Could you check a few things on this model? Use its own coordinates, in mm. A direction names the side the tool comes from. Coordinates: 2 decimals unless noted, no trailing zeros. Loops run counter-clockwise (first coordinate to the right, second up) from the corner with the lowest first, then second, coordinate; pieces in that order, holes last.
from build123d import *

# Parameters (mm, degrees)
SKETCH2_R           = 20.9
SKETCH2_R_2         = 20.4
BOSS_EXTRUDE1_DEPTH = 66
SKETCH3_R           = 20.848686735
BOSS_EXTRUDE2_DEPTH = 0.1
SKETCH4_R           = 8.6
BOSS_EXTRUDE3_DEPTH = 3.5
SKETCH5_R           = 2.4
BOSS_EXTRUDE4_DEPTH = 1.35
SKETCH7_R           = 2.4
CUT_EXTRUDE1_DEPTH  = 76.523969705
CUT_EXTRUDE6_DEPTH  = 73.316111621
CIRPATTERN2_COUNT   = 4


with BuildPart() as part:
    # Sketch2 → Boss-Extrude1 (new body)
    with BuildSketch(Plane(origin=(0, 0, 0), x_dir=(1, 0, 0), z_dir=(0, 1, 0))):
        with Locations(Location((0, 0, 0), (0, 0, 270))):
            Circle(SKETCH2_R)
        with Locations(Location((0, 0, 0), (0, 0, 270))):
            Circle(SKETCH2_R_2, mode=Mode.SUBTRACT)
    extrude(amount=BOSS_EXTRUDE1_DEPTH)

    # Sketch3 → Boss-Extrude2 (add)
    with BuildSketch(Plane(origin=(0, 0, 0), x_dir=(1, 0, 0), z_dir=(0, 1, 0))):
        Circle(SKETCH3_R)
    extrude(amount=BOSS_EXTRUDE2_DEPTH)

    # Sketch4 → Boss-Extrude3 (add)
    with BuildSketch(Plane(origin=(0, 0, 0), x_dir=(1, 0, 0), z_dir=(0, 1, 0))):
        with Locations(Location((0.271248052, 0, 0), (0, 0, 270))):
            Circle(SKETCH4_R)
    extrude(amount=-BOSS_EXTRUDE3_DEPTH)

    # Sketch5 → Boss-Extrude4 (add)
    with BuildSketch(Plane.XZ.offset(3.5)):
        with Locations((0.36166407, 0)):
            Circle(SKETCH5_R)
    extrude(amount=-BOSS_EXTRUDE4_DEPTH)

    # Sketch7 → Cut-Extrude1 (cut, through all)
    with BuildSketch(Plane.XZ.offset(3.5)):
        with Locations(Location((0.271248052, 0, 0), (0, 0, 270))):
            Circle(SKETCH7_R)
    extrude(amount=-CUT_EXTRUDE1_DEPTH, mode=Mode.SUBTRACT)

    # Sketch15 → Cut-Extrude6 (cut, through all)
    with BuildSketch(Plane(origin=(0, 0, 0), x_dir=(0, 0, -1), z_dir=(1, 0, 0))):
        with BuildLine():
            Line((-2.657246102, 51), (9.342753898, 51))
            ThreePointArc((9.342753898, 51), (12.842753898, 47.5), (9.342753898, 44))
            Line((9.342753898, 44), (-2.657246102, 44))
            ThreePointArc((-2.657246102, 44), (-6.157246102, 47.5), (-2.657246102, 51))
        make_face()
    cut_extrude6 = extrude(amount=-CUT_EXTRUDE6_DEPTH, mode=Mode.SUBTRACT)

    # CirPattern2: Cut-Extrude6 ×4 about axis
    cirpattern2_axis = Axis((0, 66, 0), (0, -1, 0))
    for i in range(1, CIRPATTERN2_COUNT):
        add(cut_extrude6.rotate(cirpattern2_axis, i * 360 / CIRPATTERN2_COUNT), mode=Mode.SUBTRACT)


solid = part.part
1) Will these pins go through, and if not, where does the flat tip stop? pin 1 (1 mm diameter, centred on x = -4, z = 0, fed in from +Y); pin 2 (5 mm diameter, centred on x = 2, y = 46, fed in from +Z); pin 3 (1.4 mm diameter, centred on x = 6.5, z = -19, fed in from -Y).
2) If I drill on L1, parallel to X at y = -2.2, z = 0; L2, parallel to X at y = 52, z = 0, over which ranges is the centre line in solid material (lowest first)?
3) Imagine slicing it at B-B on x = -4. List the corners of the cut face in (y, z) for me.
4) Imagine slicing it at C-C on y = 47.5. List the corners of the cut face in (x, z) for me.
5) Imagine slicing it at A-A on z = 0. List the corners of the cut face in (x, y) for me.
6) We'd pull the mould along X, two halves only. Please class faces 5 (the cylindrical face through (0.65, -1.73, -8.59)), 6 (the cylindrical face through (12.822, 47.119, -16.193)), 7 (the flat face through (-20.2, 51, -3.8)): released by +X, released by -X, zero draft, split by the parting line, or undercut.
7) Imagine slicing it at D-D on y = 5. List the corners of the cut face in (x, z) for me.
8) For faces 1 (the cylindrical face through (-16.193, 47.119, -12.822)), 2 (the cylindrical face through (-12.4, 32.6, -16.2)), 3 (the flat face through (-20, 66, 5)), 4 (the cylindrical face through (-12.822, 47.119, 16.193)), which set-ups out of +Z, -Z, +X, -X, +Y, -Y let a thin tool reach every point of the face, with its end or its side?
Solved:
1. pin 1: stops at y = 0.1
1. pin 2: stops at z = 20.89
1. pin 3: stops at y = 0
2. L1: x = -8.33 to -2.13, 2.67 to 8.87
2. L2: x = -20.9 to -20.4, 20.4 to 20.9
3. outline: (-3.5, -7.46) - (0, -7.46) - (0, -20.51) - (44.27, -20.51) - (44.27, -20) - (0.1, -20) - (0.1, 20) - (44, 20) - (44, 20.51) - (0, 20.51) - (0, 7.46) - (-3.5, 7.46) - close; (50.73, -20.51) - (66, -20.51) - (66, -20) - (50.73, -20) - close; (51, 20) - (66, 20) - (66, 20.51) - (51, 20.51) - close
4. outline: (-19.97, 6.16) - (-19.45, 6.16) arc R20.4 cw to (-12.84, 15.85) - (-12.84, 16.49) arc R20.9 ccw to start; (-16.49, -12.84) arc R20.9 ccw to (-6.16, -19.97) - (-6.16, -19.45) arc R20.4 cw to (-15.85, -12.84) - close; (6.16, 19.45) arc R20.4 cw to (15.85, 12.84) - (16.49, 12.84) arc R20.9 ccw to (6.16, 19.97) - close; (12.84, -16.49) arc R20.9 ccw to (19.97, -6.16) - (19.45, -6.16) arc R20.4 cw to (12.84, -15.85) - close
5. outline: (-20.9, 0) - (-8.33, 0) - (-8.33, -3.5) - (-2.13, -3.5) - (-2.13, 0.1) - (-20.4, 0.1) - (-20.4, 44) - (-20.9, 44) - close; (-20.9, 51) - (-20.4, 51) - (-20.4, 66) - (-20.9, 66) - close; (2.67, -3.5) - (8.87, -3.5) - (8.87, 0) - (20.9, 0) - (20.9, 44) - (20.4, 44) - (20.4, 0.1) - (2.67, 0.1) - close; (20.4, 51) - (20.9, 51) - (20.9, 66) - (20.4, 66) - close
6. face 5: split by the parting line
6. face 6: undercut
6. face 7: zero draft
7. outline: circle Ø41.8 at (0, 0); hole circle Ø40.8 at (0, 0)
8. face 1: -X
8. face 2: +Y
8. face 3: +Z, -Z, +X, -X, +Y
8. face 4: +Z
